from build123d import *

# Parameters (mm, degrees)
F0_R     = 10.0595284502
F1_DEPTH = 12.7
F2_R     = 5.7785
F2_R_2   = 4.1275
F3_DEPTH = 19.05


# Not quite as in the source:
# - a fillet or chamfer that OpenCascade refuses, or shapes differently, is made with other operations: its cross-section is extruded or revolved along the edge and cut away or added


with BuildPart() as f1:
    # F0 (on Top) → F1 (new body)
    with BuildSketch(Plane.XY):
        Circle(F0_R)
    extrude(amount=F1_DEPTH)

    # F2 (on face) → F3 (join)
    with BuildSketch(Plane.XY.offset(12.7)):
        Circle(F2_R)
        Circle(F2_R_2, mode=Mode.SUBTRACT)
    extrude(amount=F3_DEPTH)

    # F4: chamfer of 3.048 x 1.7597636205 on 1 edges, made by hand

    # F4_s1 → F4_t2 (revolve, cut)
    with BuildSketch(Plane.XZ):
        Polygon((5.8872636205, 31.75), (4.1275, 28.702), (4.1275, 31.75), align=None)
    revolve(axis=Axis((0, 0, 31.75), (0, 0, 1)), mode=Mode.SUBTRACT)


solid = f1.part
Can you work these out from the model? Positions are in its coordinate system, mm. A direction names the side the tool comes from. Give positions to 0.01 mm unless a question says otherwise; leave off trailing zeros. Order: outer loops, then holes, each group sorted by start corner. A loop starts at its lowest first (then second) coordinate and runs counter-clockwise, first axis right, second up. Notation, with made-up numbers: M -11,2.5 L 25,2.5 A12 cw 25,20.5 Z; hole C 62,29.5 d8. An arc over 180 degrees is marked long. Use a Markdown table: item, result. Add a question column.
Item 1: Suppose I cut it at C-C (z = 10.5). List the corners of the cut face in (x, y) for me.
Item 2: Suppose I cut it at A-A (x = 0). List the corners of the cut face in (y, z) for me.
Item 3: If I drill on L1, parallel to Y at x = 0, z = 18; L2, parallel to Z at x = -4.75, y = 6; L3, parallel to X at y = 1.25, z = 21, over which ranges is the centre line in solid material (lowest first)? Write a range as [from, to].
Item 4: Will these pins go through, and if not, where does the flat tip stop? pin 1 (6 mm diameter, centred on x = 6, z = 27.5, fed in from -Y); pin 2 (1.5 mm diameter, centred on x = 4, z = 10.5, fed in from +Y); pin 3 (1.5 mm diameter, centred on x = -0.5, z = 16.5, fed in from -Y).
Item 5: We'd pull the mould along X, two halves only. Please class faces 3 (the cylindrical face through (3.11, 4.87, 22)), 4 (the flat face through (0, 0, 0)), 5 (the flat face through (0, 0, 12.7)): +X half, -X half, draft (parallel to the pull), parting line (faces both ways), or undercut.
Item 6: For faces 1 (the cylindrical face through (-2.18, -9.82, 6.26)), 2 (the cylindrical face through (3.937, 1.24, 20.589)), which set-ups out of +Z, -Z, +X, -X, +Y, -Y let a thin tool reach every point of the face, with its end or its side?
Item 7: Suppose I cut it at D-D (z = 28). List the corners of the cut face in (x, y) for me (1 decimal), then the cut area to 3 significant figures.
Answer sheet:
| question | item | result |
|---|---|---|
| 1 | outline | C 0,0 d20.12 |
| 2 | outline | M -10.06,0 L 10.06,0 L 10.06,12.7 L 5.78,12.7 L 5.78,31.56 L 4.13,28.7 L 4.13,12.7 L -4.13,12.7 L -4.13,28.7 L -5.78,31.56 L -5.78,12.7 L -10.06,12.7 Z |
| 3 | L1 | y = [-5.78, -4.13], [4.13, 5.78] |
| 3 | L2 | z = [0, 12.7] |
| 3 | L3 | x = [-5.64, -3.93], [3.93, 5.64] |
| 4 | pin 1 | stops at y = -4.94 |
| 4 | pin 2 | stops at y = 9.52 |
| 4 | pin 3 | stops at y = -5.78 |
| 5 | face 3 | parting line |
| 5 | face 4 | draft |
| 5 | face 5 | undercut |
| 6 | face 1 | +Z, -Z |
| 6 | face 2 | +Z |
| 7 | outline | C 0,0 d11.6; hole C 0,0 d8.3 |
| 7 | area | 51.4 mm² |
